The listing builds one solid part. Answer for the finished solid, in the listing's coordinates (mm). A direction names the side the tool comes from. Give positions to 0.01 mm unless a question says otherwise; leave off trailing zeros. Order: outer loops, then holes, each group sorted by start corner. A loop starts at its lowest first (then second) coordinate and runs counter-clockwise, first axis right, second up. Notation, with made-up numbers: (56, 37.25) - (109, 37.25) arc R15 ccw to (109, 43.25) - close; hole circle Ø8 at (-39.75, -15.5). An arc over 180 degrees is marked (long way). Use a Markdown table: item, result. Add a question column.
1) The mould has two halves that part along Z. Classify faces 1 (the face through (2, -1, -26)), 2 (the face through (0.99, -13.25, -3.78)), 3 (the face through (6, 3, -18.927)): released by +Z, released by -Z, zero draft, split by the parting line, or undercut.
2) Find section C-C, the plane z = -10.5. Determine the outline of the cut face in (x, y).
3) Flat-ended cylindrical pins translate along their axes: pin 1 (4 mm diameter, centred on y = -2, z = -46, fed in from -X); pin 2 (2 mm diameter, centred on x = 4.5, y = 13, fed in from -Z) (3 decimals); pin 3 (3 mm diameter, centred on y = -6, z = -6, fed in from +X); pin 4 (6 mm diameter, centred on x = 8, y = -5, fed in from +Z). Find the tip coordinate at first contact, or state that the pin passes through.
4) For faces 4 (the face through (6, 3, -35.625)), 5 (the face through (6, 3.651, -27)), 6 (the face through (6, 12.732, -8)), determine the directions among +Z, -Z, +X, -X, +Y, -Y from which every point of the face is accessible in a straight line to the end or side of a thin tool.
5) Find section A-A, the plane x = 4. Determine the outline of the cut face in (y, z) (3 decimals), plus the area to 3 significant figures.
6) Find section B-B, the plane z = -47.3. Determine the outline of the cut face in (x, y).
7) Straight lines are drawn through the part: line 1 (Y direction, x = 0.9, z = -47.3); line 2 (Y direction, x = 1.25, z = -10.5); line 3 (Z direction, x = 3.75, y = 2.5) (3 decimals). For each, find the intervals that lie inside material, in ascending order.
8) Find section D-D, the plane y = 0.5. Determine the outline of the cut face in (x, z).
from build123d import *

# Parameters (mm, degrees)
SKETCH1_W           = 52.3
SKETCH1_H           = 32.007
SKETCH1_R           = 1
BOSS_EXTRUDE1_DEPTH = 2
SKETCH1_3_W         = 15.625
SKETCH1_3_H         = 2
SKETCH1_3_W_2       = 16.698
BOSS_EXTRUDE2_DEPTH = 10


with BuildPart() as part:
    # Sketch1 → Boss-Extrude1 (new body)
    with BuildSketch(Plane(origin=(0, 0, 0), x_dir=(0, 0, -1), z_dir=(1, 0, 0))):
        with Locations((26.15, -1.27147436)):
            Rectangle(SKETCH1_W, SKETCH1_H)
        with Locations((4, -12.27497436)):
            Circle(SKETCH1_R, mode=Mode.SUBTRACT)
        with Locations((10.5, -12.27497436)):
            Circle(SKETCH1_R, mode=Mode.SUBTRACT)
        with Locations((47.3, -9.8)):
            Circle(SKETCH1_R, mode=Mode.SUBTRACT)
        with Locations((47.3, -3.3)):
            Circle(SKETCH1_R, mode=Mode.SUBTRACT)
    extrude(amount=BOSS_EXTRUDE1_DEPTH)

    # Sketch1<3> → Boss-Extrude2 (add)
    with BuildSketch(Plane(origin=(0, 0, 0), x_dir=(0, 0, -1), z_dir=(1, 0, 0))):
        with Locations((7.8125, 13.73202564)):
            Rectangle(SKETCH1_3_W, SKETCH1_3_H)
        with Locations((27.276, 2.651)):
            Rectangle(SKETCH1_3_W_2, SKETCH1_3_H)
        with Locations((27.276, -2.651)):
            Rectangle(SKETCH1_3_W_2, SKETCH1_3_H)
    extrude(amount=BOSS_EXTRUDE2_DEPTH)


solid = part.part
The answers:
| question | item | result |
|---|---|---|
| 1 | face 1 | zero draft |
| 1 | face 2 | undercut |
| 1 | face 3 | released by +Z |
| 2 | outline | (0, -17.27) - (2, -17.27) - (2, -13.27) - (0, -13.27) - close; (0, -11.27) - (2, -11.27) - (2, 12.73) - (10, 12.73) - (10, 14.73) - (0, 14.73) - close |
| 3 | pin 1 | x = 0 |
| 3 | pin 2 | z = -15.625 |
| 3 | pin 3 | x = 2 |
| 3 | pin 4 | z = -18.93 |
| 4 | face 4 | -Z, +X, +Y, -Y |
| 4 | face 5 | +Z, -Z, +X, +Y |
| 4 | face 6 | +Z, -Z, +X, -Y |
| 5 | outline | (-3.651, -35.625) - (-1.651, -35.625) - (-1.651, -18.927) - (-3.651, -18.927) - close; (1.651, -35.625) - (3.651, -35.625) - (3.651, -18.927) - (1.651, -18.927) - close; (12.732, -15.625) - (14.732, -15.625) - (14.732, 0) - (12.732, 0) - close |
| 5 | area | 98.0 mm2 |
| 6 | outline | (0, -17.27) - (2, -17.27) - (2, -10.8) - (0, -10.8) - close; (0, -8.8) - (2, -8.8) - (2, -4.3) - (0, -4.3) - close; (0, -2.3) - (2, -2.3) - (2, 14.73) - (0, 14.73) - close |
| 7 | line 1 | -17.27 to -10.8, -8.8 to -4.3, -2.3 to 14.73 |
| 7 | line 2 | -17.27 to -13.27, -11.27 to 14.73 |
| 7 | line 3 | -35.625 to -18.927 |
| 8 | outline | (0, -52.3) - (2, -52.3) - (2, 0) - (0, 0) - close |
